Could you check a few things on this drawing? It's one solid part, dimensions in mm from its lowest x, y, z. Coordinates: 2 decimals unless noted, no trailing zeros. Write each loop counter-clockwise with the first axis right and the second up, starting at its lowest first coordinate (ties: lowest second). Pieces come first, ordered by that corner, then holes. Notation, with made-up numbers: (-4, 31) - (6, 31) arc R18 cw to (6, 53) - close; hole circle Ø2 at (8.25, 88.5). An arc over 180 degrees is marked (long way). Answer as a JSON object with one key per item and string values. Group by question number.
1) Please list where this line runs through material, in increasing order: line 1 along Z through (x, y) = (127.5, 8.25).
2) If we section it at A-A (x = 308.5): Write out the boundary of the cut face in (y, z).
3) Will these pins go through, and if not, where does the flat tip stop? pin 1 Ø3 at (x, y) = (318.5, 5) entering from +Z; pin 2 Ø1 at (x, z) = (322.5, 74.5) entering from -Y; pin 3 Ø6 at (x, y) = (120, 7) entering from -Z; pin 4 Ø3 at (y, z) = (6, 378) entering from -X.
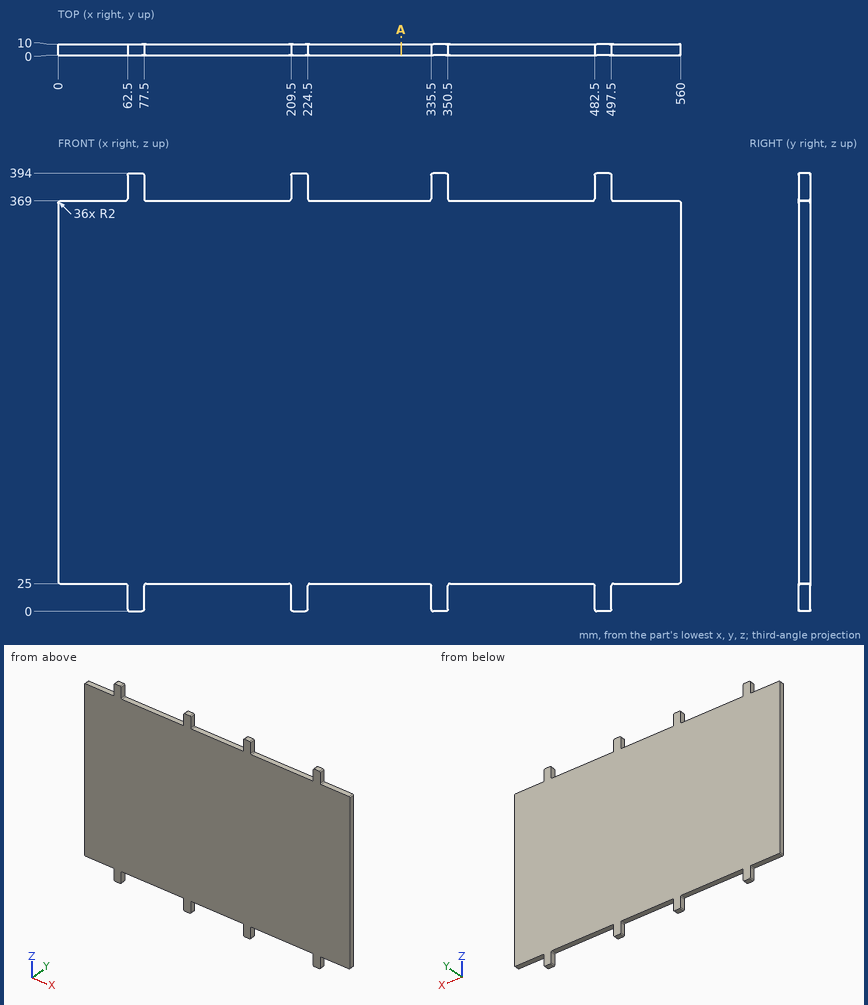
Here are the results:
{
 "1": {"line 1": "z = 25 to 369"},
 "2": {"outline": "(0, 25) - (10, 25) - (10, 369) - (0, 369) - close"},
 "3": {"pin 1": "stops at z = 369", "pin 2": "stops at y = 0", "pin 3": "stops at z = 25", "pin 4": "stops at x = 62.5"}
}
